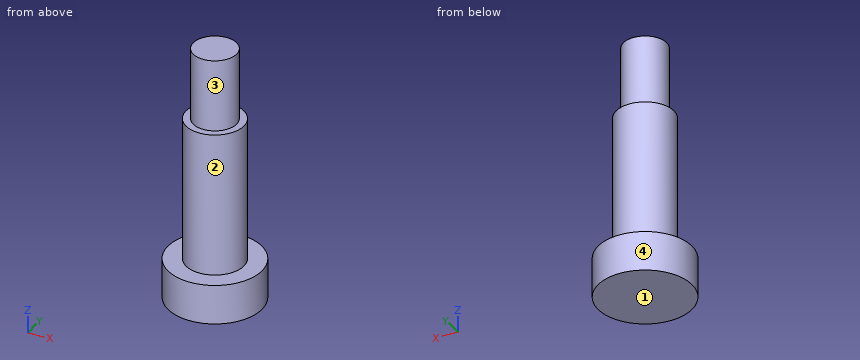
from build123d import *

# Parameters (mm, degrees)
SZKIC1_R                    = 4
DODANIE_WYCI_GNI_CIE1_DEPTH = 20
SZKIC2_R                    = 6.5
DODANIE_WYCI_GNI_CIE2_DEPTH = 5.5
SZKIC3_R                    = 3
DODANIE_WYCI_GNI_CIE3_DEPTH = 10


with BuildPart() as part:
    # Szkic1 → Dodanie-wyciągnięcie1 (new body)
    with BuildSketch(Plane.XY):
        Circle(SZKIC1_R)
    extrude(amount=DODANIE_WYCI_GNI_CIE1_DEPTH)

    # Szkic2 → Dodanie-wyciągnięcie2 (add)
    with BuildSketch(Plane(origin=(0, 0, 0), x_dir=(-1, 0, 0), z_dir=(0, 0, -1))):
        Circle(SZKIC2_R)
    extrude(amount=DODANIE_WYCI_GNI_CIE2_DEPTH)

    # Szkic3 → Dodanie-wyciągnięcie3 (add)
    with BuildSketch(Plane.XY.offset(20)):
        Circle(SZKIC3_R)
    extrude(amount=DODANIE_WYCI_GNI_CIE3_DEPTH)


solid = part.part
The model under review builds one solid part; all positions refer to its coordinate system, in mm. Face numbers are marked on the shaded views. A direction names the side the tool comes from. Round coordinates to 2 decimals unless told otherwise and drop trailing zeros. Write each loop counter-clockwise with the first axis right and the second up, starting at its lowest first coordinate (ties: lowest second). Pieces come first, ordered by that corner, then holes. Notation, with made-up numbers: M 58,32 L 117,32 A9 ccw 117,37 Z; hole C 42,54 d9. An arc over 180 degrees is marked long. Use a Markdown table: item, result. Add a question column.
Q1. To check wall thickness, follow line 1 (Z direction, x = -3.25, y = 1); line 2 (Z direction, x = -3, y = 4.5); line 3 (Y direction, x = 3.75, z = -1.5). State the ranges of each line that lie inside material, in increasing order.
Q2. We need section A-A, the plane x = 0. State the section outline as (y, z) points, plus the area to 4 significant figures.
Q3. The part is to be moulded in two halves that separate along Y. For the marked faces 1 and 2, say which applies: pulls with the +Y half, pulls with the -Y half, needs draft (parallel to the pull), parting line crosses it, or undercut.
Q4. We need section C-C, the plane z = 16.5. State the section outline as (x, y) points, plus the area to 3 significant figures.
Q5. Machinability: for the marked faces 3 and 4, which of the approach directions +Z, -Z, +X, -X, +Y, -Y give a long, thin tool a straight path to every point of the face, cutting with its end or side? Answer none if there is none.
Q6. We need section D-D, the plane z = 20.5. State the section outline as (x, y) points, plus the area to 3 significant figures.
Q7. Insertion check: pin 1 (2 mm diameter, centred on y = 3.5, z = 23.5, fed in from +X); pin 2 (1 mm diameter, centred on x = -5, z = 11.5, fed in from +Y); pin 3 (3 mm diameter, centred on x = -2, z = 12, fed in from -Y); pin 4 (1.5 mm diameter, centred on y = 3.5, z = 10.5, fed in from +X). Each pin has a flat end and moves straight along its axis. Give the tip position at first contact, or say it passes through.
Findings below:
| question | item | result |
|---|---|---|
| 1 | line 1 | z = -5.5 to 20 |
| 1 | line 2 | z = -5.5 to 0 |
| 1 | line 3 | y = -5.31 to 5.31 |
| 2 | outline | M -6.5,-5.5 L 6.5,-5.5 L 6.5,0 L 4,0 L 4,20 L 3,20 L 3,30 L -3,30 L -3,20 L -4,20 L -4,0 L -6.5,0 Z |
| 2 | area | 291.5 mm² |
| 3 | face 1 | needs draft |
| 3 | face 2 | parting line crosses it |
| 4 | outline | C 0,0 d8 |
| 4 | area | 50.3 mm² |
| 5 | face 3 | +Z |
| 5 | face 4 | +Z, -Z |
| 6 | outline | C 0,0 d6 |
| 6 | area | 28.3 mm² |
| 7 | pin 1 | stops at x = 1.66 |
| 7 | pin 2 | passes through |
| 7 | pin 3 | stops at y = -3.97 |
| 7 | pin 4 | stops at x = 2.9 |
